from build123d import *

# Parameters (mm, degrees)
F1_DEPTH  = 12.7
F3_R      = 17.4625
F4_DEPTH  = 25.4
F11_DEPTH = 25.4


with BuildPart() as f1:
    # F0 (on Right) → F1 (new body)
    with BuildSketch(Plane.YZ):
        Polygon((-27.0339550276, 20.3022155698), (-27.0339550276, 25.3198655094), (-32.0516049672, 20.3022155698), (-32.0516049672, 16.7292077094), (-6.9633552689, 16.7292077094), (-6.9633552689, 20.3022155698), (-6.9633552689, 25.3198655094), (-11.9810052086, 20.3022155698), (-11.9810052086, 25.3198655094), (-16.9986551483, 20.3022155698), (-16.9986551483, 25.3198655094), (-22.0163050879, 20.3022155698), (-22.0163050879, 25.3198655094), align=None)
    extrude(amount=F1_DEPTH)

    # F3 (on plane+point) → F4 (cut)
    with BuildSketch(Plane.XZ.offset(6.9633552689)):
        with Locations((6.3661262393, 2.0827455446)):
            Circle(F3_R)
    extrude(amount=F4_DEPTH, mode=Mode.SUBTRACT)


with BuildPart() as f5_1:
    # F5: copy of F1
    add(f1.part)


with BuildPart() as f1_1:
    # F6: moved
    add(f1.part.moved(Location((0, 26.1449348181, 0))))


with BuildPart() as f5_1_1:
    # F7: moved
    add(f5_1.part)

    # F10 (on plane+point) → F11 (cut)
    with BuildSketch(Plane.XZ.offset(6.9633552689)):
        Polygon((6.3879799563, 18.3859299868), (9.5524290794, 20.1198235154), (8.4976138382, 20.6977874041), (7.4427951975, 20.6977874041), (5.3331647151, 20.6977874041), (4.2783460745, 20.6977874041), (3.2235308333, 20.1198235154), align=None)
    extrude(amount=F11_DEPTH, mode=Mode.SUBTRACT)


with BuildPart() as f1_2:
    # F7: moved
    add(f1_1.part)


solid = f5_1_1.part
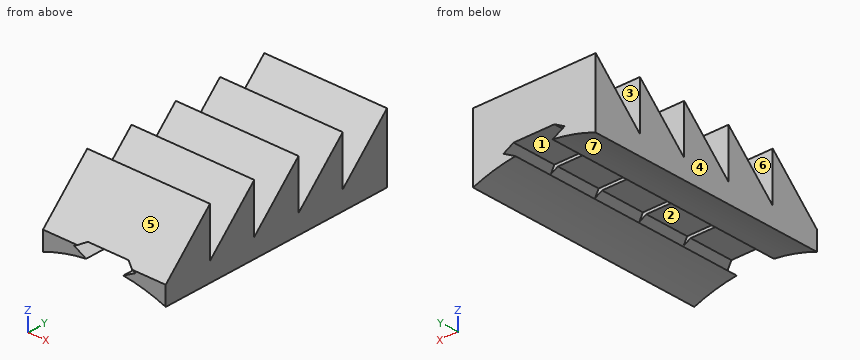
Build history of the part. All positions in model axes, mm. Face numbers are marked on the shaded views. A direction names the side the tool comes from. Give positions to 0.01 mm unless a question says otherwise; leave off trailing zeros. Order: outer loops, then holes, each group sorted by start corner. A loop starts at its lowest first (then second) coordinate and runs counter-clockwise, first axis right, second up. Notation, with made-up numbers: M 12.25,-28 L 54.25,-28 A17 ccw 54.25,-23 Z; hole C -17,2.25 d10. An arc over 180 degrees is marked long. Put each result on its own line as item: value.
Item 1: Cut at A-A on x = 7.5. Write the cut outline in (y, z).
Results are:
outline: M -31.66,20.7 L -27.03,20.7 L -27.03,25.32 Z; M -26.64,20.7 L -22.02,20.7 L -22.02,25.32 Z; M -21.62,20.7 L -17,20.7 L -17,25.32 Z; M -16.6,20.7 L -11.98,20.7 L -11.98,25.32 Z; M -11.59,20.7 L -6.96,20.7 L -6.96,25.32 Z
Item 2: Cut at D-D on x = 2. Write the cut outline in (y, z).
Results are:
outline: M -32.05,18.99 L -6.96,18.99 L -6.96,25.32 L -11.98,20.3 L -11.98,25.32 L -17,20.3 L -17,25.32 L -22.02,20.3 L -22.02,25.32 L -27.03,20.3 L -27.03,25.32 L -32.05,20.3 Z
Item 3: Drop flat-ended pins along their axis: pin 1 Ø3.5 at (x, y) = (6, -25.5) entering from -Z; pin 2 Ø1.3 at (x, y) = (7, -28.5) entering from -Z; pin 3 Ø3.5 at (x, y) = (5.5, -13.5) entering from -Z; pin 4 Ø2 at (y, z) = (-24.5, 24.5) entering from -X. Give the stop position or say it passes through.
Results are:
pin 1: z = 19.42
pin 2: z = 20.7
pin 3: z = 19.35
pin 4: through
Item 4: Which spindle directions (+Z, -Z, +X, -X, +Y, -Y) get a long thin tool onto all of the face, cutting with end or side? Do the marked faces 5, 6 and 7. Say none if no direction does.
Results are:
face 5: +Z, +X, -X, -Y
face 6: +Z, +X, -X
face 7: -Z, +Y, -Y
Item 5: Pull direction X, two halves, no side cores. Call the marked faces 1, 2, 3 and 4: +X half, -X half, draft (parallel to the pull), parting line (faces both ways), or undercut.
Results are:
face 1: undercut
face 2: undercut
face 3: draft
face 4: -X half
Item 6: Wall check: probe 1 along Y at (x, z) = (5.5, 23); probe 2 along Y at (x, z) = (11.5, 22.75); probe 3 along Z at (x, y) = (9.25, -17.75). Give the ranges that are in metal, low to high.
Results are:
probe 1: -29.35 to -27.03, -24.34 to -22.02, -19.32 to -17, -14.3 to -11.98, -9.28 to -6.96
probe 2: -29.6 to -27.03, -24.59 to -22.02, -19.57 to -17, -14.55 to -11.98, -9.53 to -6.96
probe 3: 19.31 to 19.95, 20.29 to 24.57
Item 7: Cut at C-C on y = -14.5. Write the cut outline in (x, z) (1 decimal), then the cut area to 3 significant figures.
Results are:
outline: M 0,18.3 A17.5 cw 4.5,19.4 L 3.2,20.1 L 4.3,20.7 L 8.5,20.7 L 9.6,20.1 L 8.3,19.4 A17.5 cw 12.7,18.4 L 12.7,22.8 L 0,22.8 Z
area: 40.1 mm2
Item 8: Cut at B-B on z = 21.5. Write the cut outline in (x, y).
Results are:
outline: M 0,-30.85 L 12.7,-30.85 L 12.7,-27.03 L 0,-27.03 Z; M 0,-25.84 L 12.7,-25.84 L 12.7,-22.02 L 0,-22.02 Z; M 0,-20.82 L 12.7,-20.82 L 12.7,-17 L 0,-17 Z; M 0,-15.8 L 12.7,-15.8 L 12.7,-11.98 L 0,-11.98 Z; M 0,-10.78 L 12.7,-10.78 L 12.7,-6.96 L 0,-6.96 Z
